from build123d import *

# Parameters (mm, degrees)
SKETCH1_W           = 50
SKETCH1_H           = 12.7
BOSS_EXTRUDE1_DEPTH = 50
SKETCH4_R           = 3.175
CUT_EXTRUDE2_DEPTH  = 67.154773237
SKETCH5_R           = 3.175
CUT_EXTRUDE3_DEPTH  = 30
SKETCH6_W           = 5
SKETCH6_H           = 10
BOSS_EXTRUDE3_DEPTH = 5


with BuildPart() as part:
    # Sketch1 → Boss-Extrude1 (new body)
    with BuildSketch(Plane(origin=(0, 0, 0), x_dir=(1, 0, 0), z_dir=(0, 1, 0))):
        with Locations((-16.414538776, -6.35)):
            Rectangle(SKETCH1_W, SKETCH1_H)
    extrude(amount=BOSS_EXTRUDE1_DEPTH)

    # Sketch4 → Cut-Extrude2 (cut, through all)
    with BuildSketch(Plane.XY.offset(12.7)):
        with Locations((-1.414538776, 9.5)):
            Circle(SKETCH4_R)
        with Locations((-31.414538776, 9.5)):
            Circle(SKETCH4_R)
    extrude(amount=-CUT_EXTRUDE2_DEPTH, mode=Mode.SUBTRACT)

    # Sketch5 → Cut-Extrude3 (cut)
    with BuildSketch(Plane(origin=(0, 50, 0), x_dir=(1, 0, 0), z_dir=(0, 1, 0))):
        with Locations(Location((-16.414538776, -6.35, 0), (0, 0, 270))):
            Circle(SKETCH5_R)
    extrude(amount=-CUT_EXTRUDE3_DEPTH, mode=Mode.SUBTRACT)

    # Sketch6 → Boss-Extrude3 (add)
    with BuildSketch(Plane(origin=(0, 0, 0), x_dir=(-1, 0, 0), z_dir=(0, 0, -1))):
        with Locations((16.414538776, 25)):
            Rectangle(SKETCH6_W, SKETCH6_H)
    extrude(amount=BOSS_EXTRUDE3_DEPTH)


solid = part.part
Design review of the part built by this model. Coordinates are the model's own, in mm. A direction names the side the tool comes from. Give positions to 0.01 mm unless a question says otherwise; leave off trailing zeros. Write each loop counter-clockwise with the first axis right and the second up, starting at its lowest first coordinate (ties: lowest second). Pieces come first, ordered by that corner, then holes. Notation, with made-up numbers: M 62,61 L 115,61 A24 ccw 115,90 Z; hole C 13.5,26 d4. An arc over 180 degrees is marked long. Return JSON: item names as keys, results as strings. Group by question number.
Item 1: Take a section at B-B (y = 9.5). Give the boundary of the cut face in (x, z), plus the area to 3 significant figures.
Item 2: Tool access review of faces 4 (the flat face through (-16, 20, 6)), 5 (the flat face through (-16, 30, -2)), 6 (the flat face through (-13.915, 25, -2)): name each direction out of +Z, -Z, +X, -X, +Y, -Y from which nothing blocks a thin tool from reaching the whole face with its end or side.
Item 3: The part is to be moulded in two halves that separate along X. For faces 1 (the cylindrical face through (-28.482, 8.284, 6.439)), 2 (the flat face through (8.585, 25, 6)), 3 (the flat face through (-16, 20, -2)), say which applies: pulls with the +X half, pulls with the -X half, needs draft (parallel to the pull), parting line crosses it, or undercut.
Item 4: Clearance check with flat-ended pins moving along their axes: pin 1 Ø5.5 at (x, y) = (-31.41, 9.5) entering from -Z; pin 2 Ø5.5 at (y, z) = (26.5, -3.5) entering from +X; pin 3 Ø2 at (x, y) = (-0.5, 27.5) entering from -Z; pin 4 Ø4 at (x, z) = (-16, -3.5) entering from -Y. State where each tip first meets the part, or that it passes through.
Item 5: Take a section at A-A (z = 6.35). Give the boundary of the cut face in (x, y) (3 decimals), plus the area to 3 significant figures.
Item 6: Wall thickness on line 1 along X through (y, z) = (37.75, 6.35); line 2 along Z through (x, y) = (-28.5, 20); line 3 along Y through (x, z) = (1.5, 8.25): over which ranges is each line inside the solid? List them lowest first.
Item 7: Take a section at C-C (x = -0.5). Give the boundary of the cut face in (y, z).
Item 8: Take a section at D-D (y = 23). Give the boundary of the cut face in (x, z) (3 decimals), plus the area to 3 significant figures.
Return value:
{
 "1": {"outline": "M -41.41,0 L -34.59,0 L -34.59,12.7 L -41.41,12.7 Z; M -28.24,0 L -4.59,0 L -4.59,12.7 L -28.24,12.7 Z; M 1.76,0 L 8.59,0 L 8.59,12.7 L 1.76,12.7 Z", "area": "474 mm2"},
 "2": {"face 4": "+Y", "face 5": "-Z, +X, -X, +Y", "face 6": "-Z, +X, +Y, -Y"},
 "3": {"face 1": "undercut", "face 2": "pulls with the +X half", "face 3": "needs draft"},
 "4": {"pin 1": "passes through", "pin 2": "stops at x = -13.91", "pin 3": "stops at z = 0", "pin 4": "stops at y = 20"},
 "5": {"outline": "M -41.415,0 L 8.585,0 L 8.585,50 L -13.24,50 L -13.24,20 L -19.59,20 L -19.59,50 L -41.415,50 Z; hole C -31.415,9.5 d6.35; hole C -1.415,9.5 d6.35", "area": "2,250 mm2"},
 "6": {"line 1": "x = -41.41 to -19.59, -13.24 to 8.59", "line 2": "z = 0 to 12.7", "line 3": "y = 0 to 8.24, 10.76 to 50"},
 "7": {"outline": "M 0,0 L 6.46,0 L 6.46,12.7 L 0,12.7 Z; M 12.54,0 L 50,0 L 50,12.7 L 12.54,12.7 Z"},
 "8": {"outline": "M -41.415,0 L -18.915,0 L -18.915,-5 L -13.915,-5 L -13.915,0 L 8.585,0 L 8.585,12.7 L -41.415,12.7 Z; hole C -16.415,6.35 d6.35", "area": "628 mm2"}
}
